Could you check a few things on this model? Use its own coordinates, in mm. A direction names the side the tool comes from. Coordinates: 2 decimals unless noted, no trailing zeros. Write each loop counter-clockwise with the first axis right and the second up, starting at its lowest first coordinate (ties: lowest second). Pieces come first, ordered by that corner, then holes. Notation, with made-up numbers: M -2.75,69 L 1.25,69 A32 ccw 1.25,106 Z; hole C 77.25,86 d6. An arc over 180 degrees is marked long. Answer as CSV lines item,"result". Start each with the question number.
Item 1: Suppose I cut it at D-D, the plane x = 8.25. Write out the boundary of the cut face in (y, z), and give its area (3 significant figures).
Item 2: Suppose I cut it at A-A, the plane y = -5.5. Write out the boundary of the cut face in (x, z), and give its area (3 significant figures).
Item 3: On a 3-axis mill with a long thin cutter (end or side, diameter ignored), from which of +Z, -Z, +X, -X, +Y, -Y can I reach the whole of each face in a straight line? I mean faces 4 (the flat face through (0.126, -16.425, -10.913)), 5 (the flat face through (0.126, -17.2, -8.636)). Say none if no direction works.
Item 4: Suppose I cut it at B-B, the plane x = -5. Write out the boundary of the cut face in (y, z).
Item 5: Suppose I cut it at C-C, the plane y = -16.75. Write out the boundary of the cut face in (x, z), and give its area (3 significant figures).
Item 6: If I drill on line 1 along X through (y, z) = (-4.75, -0.75); line 2 along Z through (x, y) = (7.25, -18.5); line 3 along Z through (x, y) = (-2.5, -8.75), over which ranges is the centre line in solid material (lowest first)? Write a range as [from, to].
Item 7: We'd pull the mould along X, two halves only. Please class faces 1 (the cylindrical face through (-7.691, -2.526, -1.479)), 2 (the cylindrical face through (-11.82, -2.366, -1.479)), 3 (the flat face through (0, -9, -3)): +X half, -X half, draft (parallel to the pull), parting line (faces both ways), or undercut.
Item 8: I'm going to push flat-ended pins straight in: P1, Ø6, axis at y = -18, z = -4.5, coming from the -X side; P2, Ø10, axis at x = 9, y = -3.5, coming from the -Z side; P3, Ø6, axis at y = -19.5, z = -5.5, coming from the +X side (3 decimals). Where does each tip first touch, or does it pass through?
```python
from build123d import *

# Parameters (mm, degrees)
SCHIZZO2_R               = 3
BASE_FLANGIA1_DEPTH      = 3
BORDO_FLANGIA3_DEPTH     = 17.969964774
TAGLIO_ESTRUSIONE1_DEPTH = 35.433191913


# Sheet-metal steps are written as plain solids
with BuildPart() as part:
    # Schizzo2 → Base-Flangia1 (new body)
    with BuildSketch(Plane.XY):
        with BuildLine():
            Line((-7.3, 0), (7.3, 0))
            ThreePointArc((7.3, 0), (11.777635351, -2.306133744), (12.500352166, -7.29062485))
            Line((12.500352166, -7.29062485), (8.984982387, -17.5))
            Line((8.984982387, -17.5), (-8.984982387, -17.5))
            Line((-8.984982387, -17.5), (-12.500352166, -7.29062485))
            ThreePointArc((-12.500352166, -7.29062485), (-11.777635351, -2.306133744), (-7.3, 0))
        make_face()
        with Locations((-7.3, -5.5)):
            Circle(SCHIZZO2_R, mode=Mode.SUBTRACT)
        with Locations((7.3, -5.5)):
            Circle(SCHIZZO2_R, mode=Mode.SUBTRACT)
    extrude(amount=-BASE_FLANGIA1_DEPTH)

    # Bordo-Flangia3 section (across the edge) → Bordo-Flangia3 (add)
    with BuildSketch(Plane(origin=(8.984982387, -26.21853611, -3), x_dir=(0, 0.529919264233206, 0.8480480961564254), z_dir=(-1, 0, 0))):
        with BuildLine():
            Line((-3, 8.71853611), (-3, 15))
            Line((-3, 15), (0, 15))
            Line((0, 15), (0, 8.71853611))
            ThreePointArc((0, 8.71853611), (1.81090661, 6.31538187), (4.62012024, 7.393737949))
            Line((4.62012024, 7.393737949), (7.164264529, 5.803980156))
            ThreePointArc((7.164264529, 5.803980156), (0.983994543, 3.431596782), (-3, 8.71853611))
        make_face()
    extrude(amount=BORDO_FLANGIA3_DEPTH)

    # Schizzo25 → Taglio-Estrusione1 (cut, through all)
    with BuildSketch(Plane(origin=(8.984982387, 0, 0), x_dir=(0, 0, -1), z_dir=(1, 0, 0))):
        Polygon((9.623215059, -15.619176357), (10.948788963, -13.497814667), (13.492933252, -15.08757246), (12.167359348, -17.20893415), align=None)
    extrude(amount=-TAGLIO_ESTRUSIONE1_DEPTH, mode=Mode.SUBTRACT)


solid = part.part
```
Ans:
1,outline,"M -20.41,-10.16 L -17.21,-12.17 L -15.62,-9.62 L -18.82,-7.62 A2.5 cw -17.5,-3 L -8.35,-3 L -8.35,0 L -17.5,0 A5.5 ccw Z; M -2.65,-3 L -0.08,-3 L -0.08,0 L -2.65,0 Z"
1,area,"77.5 mm^2"
2,outline,"M -12.8,-3 L -10.3,-3 L -10.3,0 L -12.8,0 Z; M -4.3,-3 L 4.3,-3 L 4.3,0 L -4.3,0 Z; M 10.3,-3 L 12.8,-3 L 12.8,0 L 10.3,0 Z"
2,area,"40.8 mm^2"
3,face 4,"-Z, +X, -X, +Y"
3,face 5,"+X, -X, +Y"
4,outline,"M -20.41,-10.16 L -17.21,-12.17 L -15.62,-9.62 L -18.82,-7.62 A2.5 cw -17.5,-3 L -7.43,-3 L -7.43,0 L -17.5,0 A5.5 ccw Z; M -3.57,-3 L 0,-3 L 0,0 L -3.57,0 Z"
5,outline,"M -9.24,-3 L 9.24,-3 L 9.24,0 L -9.24,0 Z; M -8.98,-11.43 L 8.98,-11.43 L 8.98,-8.92 L -8.98,-8.92 Z"
5,area,"101 mm^2"
6,line 1,"x = [-12.75, -10.2], [-4.4, 4.4], [10.2, 12.75]"
6,line 2,"z = [-11.36, -7.82], [-3.21, -0.09]"
6,line 3,"z = [-3, 0]"
7,face 1,"undercut"
7,face 2,"-X half"
7,face 3,"draft"
8,P1,"stops at x = -9.71"
8,P2,"stops at z = -3"
8,P3,"stops at x = 8.985"
